from build123d import *

# Parameters (mm, degrees)
SKETCH1_W           = 1.2
SKETCH1_H           = 1.2
BOSS_EXTRUDE1_DEPTH = 15
SKETCH2_R           = 2
BOSS_EXTRUDE2_DEPTH = 0.7
DOME1_FACE_RADIUS   = 2
DOME1_HEIGHT        = 0.5
FILLET1_R           = 0.1
BOSS_EXTRUDE4_DEPTH = 1.45
CUT_EXTRUDE1_DEPTH  = 1


with BuildPart() as part:
    # Sketch1 → Boss-Extrude1 (new body)
    with BuildSketch(Plane(origin=(0, 0, 0), x_dir=(1, 0, 0), z_dir=(0, 1, 0))):
        Rectangle(SKETCH1_W, SKETCH1_H)
    extrude(amount=-BOSS_EXTRUDE1_DEPTH)

    # Sketch2 → Boss-Extrude2 (add)
    with BuildSketch(Plane(origin=(0, 0, 0), x_dir=(1, 0, 0), z_dir=(0, 1, 0))):
        Circle(SKETCH2_R)
    extrude(amount=BOSS_EXTRUDE2_DEPTH)

    # Dome1: a dome of height H over a round flat face of radius A is a cap of a sphere of radius (A * A + H * H) / (2 * H)
    dome1_r = (DOME1_FACE_RADIUS * DOME1_FACE_RADIUS + DOME1_HEIGHT * DOME1_HEIGHT) / (2 * DOME1_HEIGHT)
    dome1_base = Plane((0, 0.7, 0), z_dir=(0, 1, 0))
    with Locations(dome1_base.offset(DOME1_HEIGHT - dome1_r)):
        dome1_ball = Sphere(dome1_r, mode=Mode.PRIVATE)
    add(split(dome1_ball, bisect_by=dome1_base, keep=Keep.TOP, mode=Mode.PRIVATE))

    # Fillet1
    fillet1_edges = [part.edges().sort_by_distance(p)[0] for p in [
        (1.414213562, 0.7, 1.414213562),
    ]]
    fillet(fillet1_edges, radius=FILLET1_R)

    # Sketch4 → Boss-Extrude4 (add, symmetric)
    with BuildSketch(Plane(origin=(0, 0, 0), x_dir=(0, 0, -1), z_dir=(1, 0, 0))):
        with BuildLine():
            Line((-3.400384666, -11.282296636), (-3.250384666, -11.282296636))
            add(Edge.make_bspline(
                [(-3.250384666, -11.282296636), (-3.058673713, -12.955552301), (-0.231679409, -13.114795391)],
                knots=[0, 0, 0, 1, 1, 1], degree=2))
            Line((-0.231679409, -13.114795391), (-0.231679409, -13.25444953))
            add(Edge.make_bspline(
                [(-0.231679409, -13.25444953), (-3.279731306, -13.089972513), (-3.400384666, -11.282296636)],
                knots=[0, 0, 0, 1, 1, 1], degree=2))
        make_face()
    extrude(amount=BOSS_EXTRUDE4_DEPTH, both=True)

    # Sketch5 → Cut-Extrude1 (cut)
    with BuildSketch(Plane.XY.offset(3.6)):
        with BuildLine():
            Line((-1.635819389, -12.289770392), (-1.922071278, -12.289770392))
            Line((-1.922071278, -12.289770392), (-2.158832672, -10.523660328))
            Line((-2.158832672, -10.523660328), (2.212133916, -10.523660328))
            Line((2.212133916, -10.523660328), (1.968647058, -12.372871294))
            Line((1.968647058, -12.372871294), (1.635819389, -12.289770392))
            add(Edge.make_bspline(
                [(0, -11.282296636), (1.297822629, -11.282296636), (1.635819389, -12.289770392)],
                knots=[0, 0, 0, 1, 1, 1], degree=2))
            add(Edge.make_bspline(
                [(0, -11.282296636), (-1.297822629, -11.282296636), (-1.635819389, -12.289770392)],
                knots=[0, 0, 0, 1, 1, 1], degree=2))
        make_face()
    extrude(amount=-CUT_EXTRUDE1_DEPTH, mode=Mode.SUBTRACT)


solid = part.part
Input: part model. Units: mm. Frame: model coordinates. A direction names the side the tool comes from. Give positions to 0.01 mm unless a question says otherwise; leave off trailing zeros. Order: outer loops, then holes, each group sorted by start corner. A loop starts at its lowest first (then second) coordinate and runs counter-clockwise, first axis right, second up. Notation, with made-up numbers: (-35, -17) - (4, -17) arc R22 ccw to (4, 13) - close; hole circle Ø2 at (89.5, 7.5). An arc over 180 degrees is marked (long way). Write each question's results on one line, items separated by ' | '.
Item 1: Section A-A (y = -5.75). Return loops of the section in (x, z), and give its area (3 significant figures).
A:
outline: (-0.6, -0.6) - (0.6, -0.6) - (0.6, 0.6) - (-0.6, 0.6) - close | area: 1.44 mm^2
Item 2: Draft query along Y for faces 3 (the flat face through (-0.6, -7, 0)), 4 (the flat face through (0, -15, 0)), 5 (the flat face through (1, 0, 0)), 6 (the flat face through (0, -14, 0.6)). Return one class per face: released by +Y, released by -Y, zero draft, split by the parting line, or undercut.
A:
face 3: undercut | face 4: released by -Y | face 5: undercut | face 6: zero draft
Item 3: Access query for faces 1 (the flat face through (0, -7, -0.6)), 2 (the cylindrical face through (-0.434, 0.315, 1.952)). Directions: +Z, -Z, +X, -X, +Y, -Y. A direction counts if a zero-diameter tool reaches every point of the face in a straight line with its end or side. Return the directions, or none.
A:
face 1: -Z, +X, -X, -Y | face 2: +Y
Item 4: Contact query for flat-ended pins moving along their axis: pin 1 Ø1.1 at (y, z) = (-13, 2.5) entering from -X; pin 2 Ø1.3 at (x, y) = (0, -4.5) entering from -Z; pin 3 Ø0.6 at (y, z) = (-8, 0) entering from +X. Output: stop coordinate, or through.
A:
pin 1: stops at x = -1.45 | pin 2: stops at z = -0.6 | pin 3: stops at x = 0.6
Item 5: Material intervals for line 1 along Z through (x, y) = (0.05, -11.5); line 2 along Z through (x, y) = (-0.4, -8.25), sorted ascending.
A:
line 1: z = -0.6 to 0.6, 3.21 to 3.37 | line 2: z = -0.6 to 0.6
